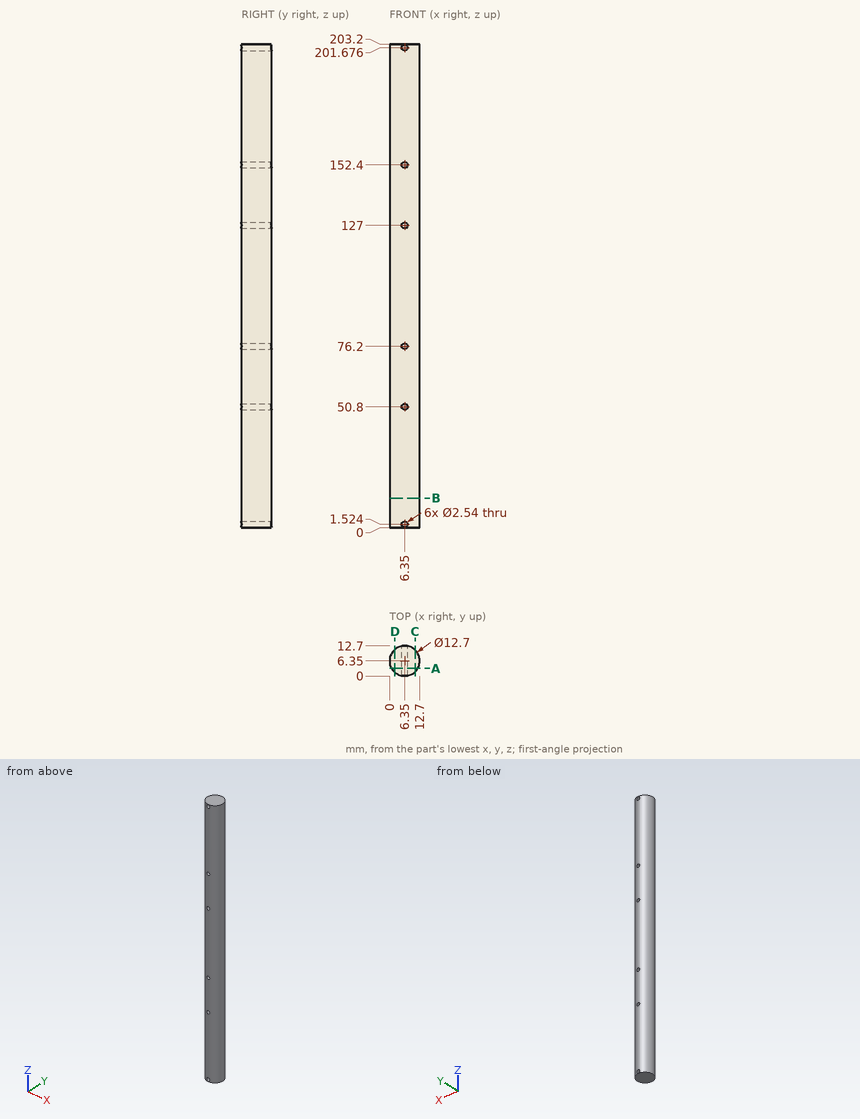
Source: three-view drawing plus pictorial views. Frame: mm from the lowest corner of the part. Give positions to 0.01 mm unless a question says otherwise; leave off trailing zeros. Order: outer loops, then holes, each group sorted by start corner. A loop starts at its lowest first (then second) coordinate and runs counter-clockwise, first axis right, second up. Notation, with made-up numbers: (84.5, 8.25) - (129.5, 8.25) arc R7 cw to (129.5, 17.25) - close; hole circle Ø8 at (85.25, 1). An arc over 180 degrees is marked (long way). Put each result on its own line as item: value.
Item 1: Section query C-C, the plane x = 10.75. Return loops of the section in (y, z), then the cut area to 3 significant figures.
Found:
outline: (1.77, 0) - (10.93, 0) - (10.93, 203.2) - (1.77, 203.2) - close
area: 1,860 mm^2
Item 2: Contact query for flat-ended pins moving along their axis: pin 1 (3 mm diameter, centred on x = 8, z = 152.5, fed in from +Y); pin 2 (5 mm diameter, centred on x = 2, z = 101, fed in from +Y); pin 3 (5 mm diameter, centred on y = 9, z = 130.5, fed in from +X). Output: stop coordinate, or through.
Found:
pin 1: stops at y = 12.67
pin 2: stops at y = 12.42
pin 3: stops at x = 12.7
Item 3: Section query B-B, the plane z = 12.5. Return loops of the section in (x, y), then the cut area to 3 significant figures.
Found:
outline: circle Ø12.7 at (6.35, 6.35)
area: 127 mm^2
Item 4: Ray query, L1, parallel to X at y = 10, z = 76; L2, parallel to Y at x = 6.75, z = 57.5; L3, parallel to X at y = 5, z = 109. Return the intervals inside material, ascending. Write a range as from..to.
Found:
L1: x = 1.15..5.1, 7.6..11.55
L2: y = 0.01..12.69
L3: x = 0.15..12.55
Item 5: Section query A-A, the plane y = 3.25. Return loops of the section in (x, z).
Found:
outline: (0.81, 0) - (11.89, 0) - (11.89, 203.2) - (0.81, 203.2) - close; hole circle Ø2.54 at (6.35, 1.52); hole circle Ø2.54 at (6.35, 50.8); hole circle Ø2.54 at (6.35, 76.2); hole circle Ø2.54 at (6.35, 127); hole circle Ø2.54 at (6.35, 152.4); hole circle Ø2.54 at (6.35, 201.68)
Item 6: Section query D-D, the plane x = 2.25. Return loops of the section in (y, z).
Found:
outline: (1.5, 0) - (11.2, 0) - (11.2, 203.2) - (1.5, 203.2) - close
